```python
from build123d import *

# Parameters (mm, degrees)
EXTRUDE_1_DEPTH        = 46.5
HOLE_WIZARD_M4_1_D     = 3.3
HOLE_WIZARD_M4_1_DEPTH = 12
HOLE_WIZARD_M4_1_TIP   = 0.991420021
SKETCH_4_R             = 2
EXTRUDE_2_DEPTH        = 6


with BuildPart() as part:
    # 草图1 → 凸台-拉伸1 (new body)
    with BuildSketch(Plane.XY):
        with BuildLine():
            Line((-1.732050808, 2.75), (1.732050808, 2.75))
            ThreePointArc((1.732050808, 2.75), (3.25, 0), (1.732050808, -2.75))
            Line((1.732050808, -2.75), (-1.732050808, -2.75))
            ThreePointArc((-1.732050808, -2.75), (-3.25, 0), (-1.732050808, 2.75))
        make_face()
    extrude(amount=EXTRUDE_1_DEPTH)

    # M4 螺纹孔1
    with Locations(Plane.XY.offset(46.5)):
        with Locations((0, 0)):
            Hole(HOLE_WIZARD_M4_1_D / 2, depth=HOLE_WIZARD_M4_1_DEPTH)
            with Locations((0, 0, -(HOLE_WIZARD_M4_1_DEPTH + HOLE_WIZARD_M4_1_TIP / 2))):  # 118° drill point
                Cone(0, HOLE_WIZARD_M4_1_D / 2, HOLE_WIZARD_M4_1_TIP, mode=Mode.SUBTRACT)

    # 草图4 → 凸台-拉伸2 (add)
    with BuildSketch(Plane(origin=(0, 0, 0), x_dir=(-1, 0, 0), z_dir=(0, 0, -1))):
        Circle(SKETCH_4_R)
    extrude(amount=EXTRUDE_2_DEPTH)


solid = part.part
```
Source: CAD feature listing. Evaluate the final solid. Frame: model axes, mm. A direction names the side the tool comes from. Give positions to 0.01 mm unless a question says otherwise; leave off trailing zeros. Write each loop counter-clockwise with the first axis right and the second up, starting at its lowest first coordinate (ties: lowest second). Pieces come first, ordered by that corner, then holes. Notation, with made-up numbers: (-14, 31.25) - (7, 31.25) arc R12 ccw to (7, 39.25) - close; hole circle Ø3 at (89, 73). An arc over 180 degrees is marked (long way). One line per item, written item: value. Start each with the question number.
Q1. Draft query along Y for faces 1 (the face through (0, -2, 46.5)), 2 (the face through (3.25, 0.05, 22.92)), 3 (the face through (-0.1, -0.3, 33.7)). Return one class per face: +Y half, -Y half, draft (parallel to the pull), parting line (faces both ways), or undercut.
Q2. Section query A-A, the plane z = 37. Return the cut outline in (x, y), then the cut area to 3 significant figures.
Q3. Set-up query: faces 4 (the face through (1.216, 1.115, 40.416)), 5 (the face through (1, 2, 0)), 6 (the face through (0, 2.75, 23)). Return all of +Z, -Z, +X, -X, +Y, -Y with unobstructed straight access to the full face (end or side cutting, diameter ignored); none if empty.
Q4. Section query B-B, the plane z = 12. Return the cut outline in (x, y).
Q5. Material intervals for probe 1 along Y at (x, z) = (0, 39); probe 2 along Z at (x, y) = (-2.5, -1.65); probe 3 along X at (y, z) = (-0.25, 38.5), sorted ascending. Write a range as from..to.
Answer:
1. face 1: draft
1. face 2: parting line
1. face 3: undercut
2. outline: (-1.73, -2.75) - (1.73, -2.75) arc R3.25 ccw to (1.73, 2.75) - (-1.73, 2.75) arc R3.25 ccw to start; hole circle Ø3.3 at (0, 0)
2. area: 22.3 mm2
3. face 4: +Z
3. face 5: -Z
3. face 6: +Z, -Z, +X, -X, +Y
4. outline: (-1.73, -2.75) - (1.73, -2.75) arc R3.25 ccw to (1.73, 2.75) - (-1.73, 2.75) arc R3.25 ccw to start
5. probe 1: y = -2.75..-1.65, 1.65..2.75
5. probe 2: z = 0..46.5
5. probe 3: x = -3.24..-1.63, 1.63..3.24
